```python
from build123d import *


with BuildPart() as f2:
    # F1 (on Front) → F2 (revolve)
    with BuildSketch(Plane.XZ):
        with BuildLine():
            Line((-24.2999375641, -2.3), (-22.4999375641, -2.3))
            ThreePointArc((-22.4999375641, -2.3), (-20.1999375641, 0), (-22.4999375641, 2.3))
            Line((-22.4999375641, 2.3), (-22.7000582963, 2.3))
            Line((-22.7000582963, 2.3), (-22.7000582963, 6.5))
            Line((-22.7000582963, 6.5), (-24.2999375641, 6.5))
            ThreePointArc((-24.2999375641, 6.5), (-24.6534909547, 6.3535533906), (-24.7999375641, 6))
            Line((-24.7999375641, 6), (-24.7999375641, 2))
            Line((-24.7999375641, 2), (-24.7999375641, -1.8))
            ThreePointArc((-24.7999375641, -1.8), (-24.6534909547, -2.1535533906), (-24.2999375641, -2.3))
        make_face()
    revolve(axis=Axis((0, 0, 0), (0, 0, 1)))


solid = f2.part
```
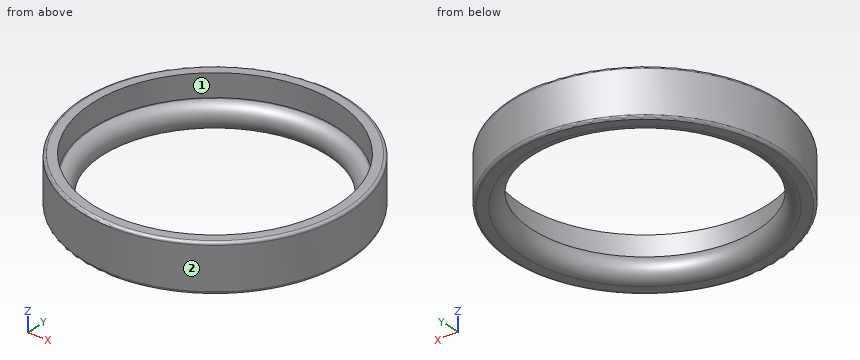
Source: CAD feature listing. Evaluate the final solid. Frame: model axes, mm. Face numbers are marked on the shaded views. Round coordinates to 2 decimals unless told otherwise and drop trailing zeros. Loops run counter-clockwise (first coordinate to the right, second up) from the corner with the lowest first, then second, coordinate; pieces in that order, holes last. Notation, with made-up numbers: M 30,67 L 68,67 A28 ccw 68,98 Z; hole C 35.25,-26 d5. An arc over 180 degrees is marked long. Use a Markdown table: item, result. Add a question column.
1. Contact query for flat-ended pins moving along their axis: P1, Ø4, axis at x = -19.5, z = -0.5, coming from the -Y side; P2, Ø5, axis at x = -9, z = 0.5, coming from the +Y side; P3, Ø5, axis at x = 18, z = 2.5, coming from the -Y side. Output: stop coordinate, or through.
2. Section query C-C on z = 4.25. Return the cut outline in (x, y), then the cut area to 3 significant figures.
3. Section query A-A on x = 0. Return the cut outline in (y, z), then the cut area to 3 significant figures.
4. Mould query, pull axis Y, two halves, no side actions, for the marked faces 1 and 2. Classes: pulls with the +Y half, pulls with the -Y half, needs draft (parallel to the pull), parting line crosses it, or undercut.
5. Line query: line 1 (X direction, y = 0, z = 5.35); line 2 (X direction, y = -6, z = 1). Output: solid intervals per line, ascending.
6. Section query D-D on z = -0.5. Return the cut outline in (x, y).
Reported:
| question | item | result |
|---|---|---|
| 1 | P1 | stops at y = -17.57 |
| 1 | P2 | stops at y = 23.93 |
| 1 | P3 | stops at y = -19.36 |
| 2 | outline | C 0,0 d49.6; hole C 0,0 d45.4 |
| 2 | area | 313 mm² |
| 3 | outline | M -24.8,-1.8 A0.5 ccw -24.3,-2.3 L -22.5,-2.3 A2.3 ccw -22.5,2.3 L -22.7,2.3 L -22.7,6.5 L -24.3,6.5 A0.5 ccw -24.8,6 Z; M 22.5,-2.3 L 24.3,-2.3 A0.5 ccw 24.8,-1.8 L 24.8,6 A0.5 ccw 24.3,6.5 L 22.7,6.5 L 22.7,2.3 L 22.5,2.3 A2.3 ccw Z |
| 3 | area | 55.2 mm² |
| 4 | face 1 | undercut |
| 4 | face 2 | parting line crosses it |
| 5 | line 1 | x = -24.8 to -22.7, 22.7 to 24.8 |
| 5 | line 2 | x = -24.06 to -19.53, 19.53 to 24.06 |
| 6 | outline | C 0,0 d49.6; hole C 0,0 d40.51 |
